```python
from build123d import *

# Parameters (mm, degrees)
SKETCH1_W           = 315.58
SKETCH1_H           = 3.175
BOSS_EXTRUDE1_DEPTH = 232.600000128
SKETCH5_W           = 3.175
SKETCH5_H           = 130.999992
CUT_EXTRUDE2_DEPTH  = 282.088108579
SKETCH8_W           = 99.68
SKETCH8_H           = 3.175
BOSS_EXTRUDE2_DEPTH = 3.175


with BuildPart() as part:
    # Sketch1 → Boss-Extrude1 (new body)
    with BuildSketch(Plane.XY):
        Rectangle(SKETCH1_W, SKETCH1_H)
    extrude(amount=BOSS_EXTRUDE1_DEPTH)

    # Sketch5 → Cut-Extrude2 (cut, symmetric)
    with BuildSketch(Plane(origin=(0, 1.5875, 0), x_dir=(1, 0, 0), z_dir=(0, 1, 0))):
        with Locations((-156.2025, -65.499996)):
            Rectangle(SKETCH5_W, SKETCH5_H)
    cut_extrude2 = extrude(amount=CUT_EXTRUDE2_DEPTH, both=True, mode=Mode.SUBTRACT)

    # Mirror1: Cut-Extrude2 across plane
    add(cut_extrude2.mirror(Plane(origin=(0, 0, 0), x_dir=(0, 0, 1), z_dir=(1, 0, 0))), mode=Mode.SUBTRACT)

    # Sketch8 → Boss-Extrude2 (add)
    with BuildSketch(Plane(origin=(0, 0, 0), x_dir=(-1, 0, 0), z_dir=(0, 0, -1))):
        Rectangle(SKETCH8_W, SKETCH8_H)
    extrude(amount=BOSS_EXTRUDE2_DEPTH)


solid = part.part
```
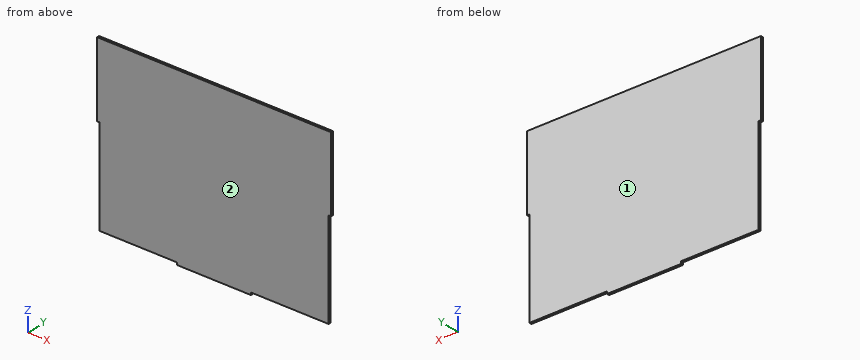
The listing builds one solid part. Answer for the finished solid, in the listing's coordinates (mm). Face numbers are marked on the shaded views. Give positions to 0.01 mm unless a question says otherwise; leave off trailing zeros. Order: outer loops, then holes, each group sorted by start corner. A loop starts at its lowest first (then second) coordinate and runs counter-clockwise, first axis right, second up. Notation, with made-up numbers: (-35.5, -10.75) -> (-8.5, -10.75) arc R22 ccw to (-8.5, 6.25) -> close; hole circle Ø2 at (5, 10). An arc over 180 degrees is marked (long way). Answer as a JSON object with one key per item and string values. Group by question number.
Item 1: Consider L1, parallel to X at y = -0.65, z = 62.5 (3 decimals); L2, parallel to Z at x = 94.5, y = 0.5. Determine where each line is inside the solid, lowest interval first. Write a range as from..to.
Item 2: Flat-ended cylindrical pins translate along their axes: pin 1 (1.6 mm diameter, centred on y = -0.5, z = -1, fed in from +X); pin 2 (1.5 mm diameter, centred on y = -1, z = 74, fed in from -X) (3 decimals); pin 3 (1.6 mm diameter, centred on x = -156.5, y = 0.5, fed in from -Z). Find the tip coordinate at first contact, or state that the pin passes through.
Item 3: Determine the mould class of the marked faces 1 and 2 for opening direction Y: pulls with the +Y half, pulls with the -Y half, needs draft (parallel to the pull), parting line crosses it, or undercut.
Item 4: The part is cut by section A-A on y = -0.05. Write down the section's boundary in (x, z) (3 decimals).
Item 5: The part is cut by section B-B on z = 55.5. Write down the section's boundary in (x, y) (1 decimal).
Result set:
{
 "1": {"L1": "-154.615..154.615", "L2": "0..232.6"},
 "2": {"pin 1": "x = 49.84", "pin 2": "x = -154.615", "pin 3": "z = 131"},
 "3": {"face 1": "pulls with the +Y half", "face 2": "pulls with the -Y half"},
 "4": {"outline": "(-157.79, 131) -> (-154.615, 131) -> (-154.615, 0) -> (-49.84, 0) -> (-49.84, -3.175) -> (49.84, -3.175) -> (49.84, 0) -> (154.615, 0) -> (154.615, 131) -> (157.79, 131) -> (157.79, 232.6) -> (-157.79, 232.6) -> close"},
 "5": {"outline": "(-154.6, -1.6) -> (154.6, -1.6) -> (154.6, 1.6) -> (-154.6, 1.6) -> close"}
}
